Autodesk Inventor part; units mm, degrees
ref_plane "Work Plane1" through (0, 0, 10) normal (0, 0, 1) x (1, 0, 0)
ref_plane "Work Plane2" through (0, 0, 10) normal (0, 0, -1) x (-1, 0, 0)
ref_plane "YZ Plane" through (0, 0, 0) normal (1, 0, 0) x (0, 1, 0)
sketch "Sketch1" plane through (0, 0, 0) normal (0, 0, 1) x (1, 0, 0)
  circle A0 centre (0, 0) radius 18.33
  arc A1 (-1.8, 7.7127) -> (-3.5788, 7.0653) centre (0, 0) ccw
  arc A2 (3.5788, 7.0653) -> (1.8, 7.7127) centre (0, 0) ccw
  arc A3 (7.3109, 3.0458) -> (6.3365, 4.7513) centre (0, 0) ccw
  arc A4 (7.5794, -2.2975) -> (7.9081, -0.4334) centre (0, 0) ccw
  arc A5 (4.3294, -6.632) -> (5.7794, -5.4152) centre (0, 0) ccw
  arc A6 (-0.9465, -7.8632) -> (0.9465, -7.8632) centre (0, 0) ccw
  arc A7 (-5.7794, -5.4152) -> (-4.3294, -6.632) centre (0, 0) ccw
  arc A8 (-6.3365, 4.7513) -> (-7.283, 3.112) centre (0, 0) ccw
  arc A9 (-7.9081, -0.4334) -> (-7.5794, -2.2975) centre (0, 0) ccw
  line L0 (-0.9465, -7.8632) -> (-2.2366, -11.4078)
  line L1 (-4.3294, -6.632) -> (-5.6195, -10.1765)
  line L2 (-5.6195, -10.1765) -> (-4.5495, -12.0298)
  line L3 (-2.2366, -11.4078) -> (-4.2475, -12.1397)
  arc A10 (-4.5495, -12.0298) -> (-4.2475, -12.1397) centre (-4.333, -11.9048) ccw
  line L4 (4.3294, -6.632) -> (5.6195, -10.1765)
  line L5 (0.9465, -7.8632) -> (2.2366, -11.4078)
  line L6 (2.2366, -11.4078) -> (4.2475, -12.1397)
  line L7 (5.6195, -10.1765) -> (4.5495, -12.0298)
  arc A11 (4.2475, -12.1397) -> (4.5495, -12.0298) centre (4.333, -11.9048) ccw
  line L8 (7.5794, -2.2975) -> (10.8461, -4.1836)
  line L9 (5.7794, -5.4152) -> (9.0461, -7.3012)
  line L10 (9.0461, -7.3012) -> (11.057, -6.5693)
  line L11 (10.8461, -4.1836) -> (11.2177, -6.291)
  arc A12 (11.057, -6.5693) -> (11.2177, -6.291) centre (10.9715, -6.3344) ccw
  line L12 (7.283, 3.112) -> (10.9978, 3.767)
  line L13 (7.9081, -0.4334) -> (11.6229, 0.2217)
  line L14 (11.6229, 0.2217) -> (12.6929, 2.0749)
  line L15 (10.9978, 3.767) -> (12.6371, 2.3914)
  arc A13 (12.6929, 2.0749) -> (12.6371, 2.3914) centre (12.4764, 2.1999) ccw
  line L16 (3.5788, 7.0653) -> (6.0034, 9.9549)
  line L17 (6.3365, 4.7513) -> (8.7612, 7.6408)
  line L18 (8.7612, 7.6408) -> (8.3896, 9.7483)
  line L19 (6.0034, 9.9549) -> (8.1434, 9.9549)
  arc A14 (8.3896, 9.7483) -> (8.1434, 9.9549) centre (8.1434, 9.7049) ccw
  line L20 (-1.8, 7.7127) -> (-1.8, 11.4848)
  line L21 (1.8, 7.7127) -> (1.8, 11.4848)
  line L22 (1.8, 11.4848) -> (0.1607, 12.8603)
  line L23 (-1.8, 11.4848) -> (-0.1607, 12.8603)
  arc A15 (0.1607, 12.8603) -> (-0.1607, 12.8603) centre (0, 12.6688) ccw
  line L24 (-6.3365, 4.7513) -> (-8.7612, 7.6408)
  line L25 (-3.5788, 7.0653) -> (-6.0034, 9.9549)
  line L26 (-6.0034, 9.9549) -> (-8.1434, 9.9549)
  line L27 (-8.7612, 7.6408) -> (-8.3896, 9.7483)
  arc A16 (-8.1434, 9.9549) -> (-8.3896, 9.7483) centre (-8.1434, 9.7049) ccw
  line L28 (-7.9081, -0.4334) -> (-11.6229, 0.2217)
  line L29 (-7.283, 3.112) -> (-10.9978, 3.767)
  line L30 (-10.9978, 3.767) -> (-12.6371, 2.3914)
  line L31 (-11.6229, 0.2217) -> (-12.6929, 2.0749)
  arc A17 (-12.6371, 2.3914) -> (-12.6929, 2.0749) centre (-12.4764, 2.1999) ccw
  line L32 (-5.7794, -5.4152) -> (-9.0461, -7.3012)
  line L33 (-7.5794, -2.2975) -> (-10.8461, -4.1836)
  line L34 (-10.8461, -4.1836) -> (-11.2177, -6.291)
  line L35 (-9.0461, -7.3012) -> (-11.057, -6.5693)
  arc A18 (-11.2177, -6.291) -> (-11.057, -6.5693) centre (-10.9715, -6.3344) ccw
  arc A19 (-0.9465, -7.8632) -> (0.9465, -7.8632) centre (0, 0) ccw
  arc A20 (4.3294, -6.632) -> (5.7794, -5.4152) centre (0, 0) ccw
  arc A21 (7.5794, -2.2975) -> (7.9081, -0.4334) centre (0, 0) ccw
  arc A22 (7.283, 3.112) -> (6.3365, 4.7513) centre (0, 0) ccw
  arc A23 (3.5788, 7.0653) -> (1.8, 7.7127) centre (0, 0) ccw
  arc A24 (-1.8, 7.7127) -> (-3.5788, 7.0653) centre (0, 0) ccw
  arc A25 (-6.3365, 4.7513) -> (-7.283, 3.112) centre (0, 0) ccw
  arc A26 (-7.9081, -0.4334) -> (-7.5794, -2.2975) centre (0, 0) ccw
  arc A27 (-5.7794, -5.4152) -> (-4.3294, -6.632) centre (0, 0) ccw
  point P0 (-2.306, -11.394)
  point P1 (-5.5574, -10.2106)
  dimension "d58" = 0.25
  dimension "d61" = 360
ref_plane "Work Plane1" through (0, 0, 10) normal (0, 0, 1) x (1, 0, 0)
sketch "Sketch2" plane through (0, 0, 10) normal (0, 0, 1) x (1, 0, 0)
  circle A0 centre (0, 0) radius 34.925
  circle A1 centre (0, 23.8125) radius 3.302
  circle A2 centre (-20.6222, 11.9063) radius 3.302
  circle A3 centre (-20.6222, -11.9062) radius 3.302
  circle A4 centre (0, -23.8125) radius 3.302
  circle A5 centre (20.6222, -11.9063) radius 3.302
  circle A6 centre (20.6222, 11.9062) radius 3.302
  dimension "d42" = 69.85
  dimension "d44" = 6.604
  dimension "d47" = 360
extrude "Extrusion2" add sketch "Sketch2" along normal blind 6.35
ref_plane "Work Plane2" through (0, 0, 10) normal (0, 0, -1) x (-1, 0, 0)
extrude "Extrusion4" add sketch "Sketch1" along normal up to surface (10 mm away)
sketch "Sketch4" plane through (0, 0, 10) normal (0, 0, -1) x (-1, 0, 0)
  circle A0 centre (0, 0) radius 4.5
  dimension "d65" = 9
extrude "Extrusion5" cut sketch "Sketch4" against normal blind 10
fillet "Fillet1" radius 2 1 edges at (-18.33, 0, 10)
sketch "Sketch6" plane through (0, 0, 16.35) normal (0, 0, 1) x (1, 0, 0)
  circle A0 centre (0, 0) radius 34.925
  circle A1 centre (0, -23.8125) radius 3.302
  circle A2 centre (0, -23.8125) radius 3.302
  circle A3 centre (20.6222, -11.9063) radius 3.302
  circle A4 centre (20.6222, 11.9062) radius 3.302
  circle A5 centre (0, 23.8125) radius 3.302
  circle A6 centre (-20.6222, 11.9063) radius 3.302
  circle A7 centre (-20.6222, -11.9062) radius 3.302
  dimension "d77" = 360
extrude "Extrusion7" add sketch "Sketch6" along normal blind 6.05
sketch "Sketch7" plane through (0, 0, 16.35) normal (0, 0, -1) x (-1, 0, 0)
  circle A0 centre (0, 0) radius 4.5
extrude "Extrusion8" cut sketch "Sketch7" against normal up to surface (6.05 mm away)
chamfer "Chamfer1" distance 2 angle 45 1 edges at (4.5, 0, 10)
properties part number "Window Motor Adapter"
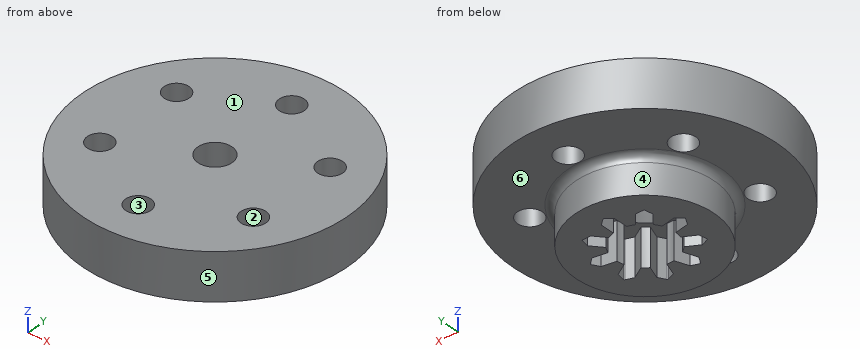
Part model, mm, in its own coordinate system. Face numbers are marked on the shaded views. A direction names the side the tool comes from. Give positions to 0.01 mm unless a question says otherwise; leave off trailing zeros. Order: outer loops, then holes, each group sorted by start corner. A loop starts at its lowest first (then second) coordinate and runs counter-clockwise, first axis right, second up. Notation, with made-up numbers: M 3.5,41.25 L 48.5,41.25 A15 cw 48.5,68.25 Z; hole C 59,-39 d2. An arc over 180 degrees is marked long. Use a Markdown table: item, result. Add a question column.
(1) Saw through at C-C, the plane y = 30. Give the cut face in (x, z), and give its area (3 significant figures).
(2) 3-axis set-ups, long thin cutter, end or side, ignore diameter. For the marked faces 5 and 6: which of +Z, -Z, +X, -X, +Y, -Y reach the whole face in a straight line?
(3) Saw through at A-A, the plane z = 18.25. Give the number of separate pieces and of enclosed holes in the cut face, and give its area (3 significant figures).
(4) Probe line 1 along Y through (x, z) = (0, 19) (1 decimal); line 2 along Y through (x, z) = (2, 21.75); line 3 along Z through (x, y) = (5, 23). List the from-to ranges inside material, lowest first. Write a range as [from, to].
(5) Drop flat-ended pins along their axis: P1, Ø7.5, axis at x = -3, y = 0, coming from the -Z side; P2, Ø6, axis at x = 20.62, y = -11.91, coming from the -Z side; P3, Ø0.6, axis at x = -7.5, z = 6, coming from the -Y side; P4, Ø2.5, axis at x = 7.5, z = 4.5, coming from the -Y side. Give the stop position or say it passes through.
(6) Mould opens along Y. For the marked faces 1, 2, 3 and 4 say: +Y half, -Y half, draft (parallel to the pull), parting line (faces both ways), or undercut.
Answer key:
| question | item | result |
|---|---|---|
| 1 | outline | M -17.88,10 L 17.88,10 L 17.88,22.4 L -17.88,22.4 Z |
| 1 | area | 443 mm^2 |
| 2 | face 5 | +Z, -Z |
| 2 | face 6 | -Z |
| 3 | separate pieces | 1 |
| 3 | enclosed holes | 7 |
| 3 | area | 3,560 mm^2 |
| 4 | line 1 | [-34.9, -27.1], [-20.5, -4.5], [4.5, 20.5], [27.1, 34.9] |
| 4 | line 2 | [-34.87, -26.44], [-21.19, -4.03], [4.03, 21.19], [26.44, 34.87] |
| 4 | line 3 | [10, 22.4] |
| 5 | P1 | z = 10 |
| 5 | P2 | through |
| 5 | P3 | y = -16.86 |
| 5 | P4 | y = -17.23 |
| 6 | face 1 | draft |
| 6 | face 2 | undercut |
| 6 | face 3 | undercut |
| 6 | face 4 | parting line |
